For this review, take the finished solid that the model builds, in its own axes (mm). A direction names the side the tool comes from. Give positions to 0.01 mm unless a question says otherwise; leave off trailing zeros. Order: outer loops, then holes, each group sorted by start corner. A loop starts at its lowest first (then second) coordinate and runs counter-clockwise, first axis right, second up. Notation, with made-up numbers: (56, -2.5) - (66, -2.5) arc R12 ccw to (66, 8.5) - close; hole circle Ø3 at (36.5, 66.25). An arc over 180 degrees is marked (long way). One line per item, written item: value.
```python
from build123d import *

# Parameters (mm, degrees)
F0_W     = 76.2
F0_H     = 152.4
F1_DEPTH = 25.4
F2_W     = 33.02
F2_H     = 21.1666666667
F3_DEPTH = 22.86
F4_DEPTH = 22.86
F5_DEPTH = 22.86


# Not quite as in the source:
# - a feature names something its author has since deleted; it is built from what else it names


with BuildPart() as f1:
    # F0 (on Front) → F1 (new body)
    with BuildSketch(Plane.XZ):
        Rectangle(F0_W, F0_H)
    extrude(amount=F1_DEPTH)

    # F2 (on face) → F3 (cut)
    with BuildSketch(Plane.XZ.offset(25.4)):
        with Locations((-18.2778849706, 54.3725310351)):
            Rectangle(F2_W, F2_H)
    extrude(amount=-F3_DEPTH, mode=Mode.SUBTRACT)

    # F2 (on face) → F4 (cut)
    with BuildSketch(Plane.XZ.offset(25.4)):
        with Locations((19.8221150294, 54.3725310351)):
            Rectangle(F2_W, F2_H)
        with Locations((-19.05, 28.5166088839)):
            Rectangle(F2_W, F2_H)
        with Locations((-18.5682759488, -3.211494873)):
            Rectangle(F2_W, F2_H)
        with Locations((19.5317240512, -3.211494873)):
            Rectangle(F2_W, F2_H)
    extrude(amount=-F4_DEPTH, mode=Mode.SUBTRACT)

    # F2 (on face) → F5 (cut)
    with BuildSketch(Plane.XZ.offset(25.4)):
        with Locations((19.05, 28.5166088839)):
            Rectangle(F2_W, F2_H)
    extrude(amount=-F5_DEPTH, mode=Mode.SUBTRACT)


solid = f1.part
```
(1) Wall thickness on line 1 (Z direction, x = -34, y = -11); line 2 (X direction, y = -9.25, z = 23); line 3 (X direction, y = -16, z = 6.5): over which ranges is each line inside the solid? List them lowest first. Write a range as from..to.
Answers below:
line 1: z = -76.2..-13.79, 7.37..17.93, 39.1..43.79, 64.96..76.2
line 2: x = -38.1..-35.56, -2.54..2.54, 35.56..38.1
line 3: x = -38.1..-35.08, -2.06..3.02, 36.04..38.1
(2) Take a section at C-C (x = 17). Write out the cut boundary in (y, z).
Answers below:
outline: (-25.4, -76.2) - (0, -76.2) - (0, 76.2) - (-25.4, 76.2) - (-25.4, 64.96) - (-2.54, 64.96) - (-2.54, 43.79) - (-25.4, 43.79) - (-25.4, 39.1) - (-2.54, 39.1) - (-2.54, 17.93) - (-25.4, 17.93) - (-25.4, 7.37) - (-2.54, 7.37) - (-2.54, -13.79) - (-25.4, -13.79) - close
(3) Take a section at A-A (y = -8.5). Write out the cut boundary in (x, z).
Answers below:
outline: (-38.1, -76.2) - (38.1, -76.2) - (38.1, 76.2) - (-38.1, 76.2) - close; hole (-35.56, 17.93) - (-2.54, 17.93) - (-2.54, 39.1) - (-35.56, 39.1) - close; hole (-35.08, -13.79) - (-2.06, -13.79) - (-2.06, 7.37) - (-35.08, 7.37) - close; hole (-34.79, 43.79) - (-1.77, 43.79) - (-1.77, 64.96) - (-34.79, 64.96) - close; hole (2.54, 17.93) - (35.56, 17.93) - (35.56, 39.1) - (2.54, 39.1) - close; hole (3.02, -13.79) - (36.04, -13.79) - (36.04, 7.37) - (3.02, 7.37) - close; hole (3.31, 43.79) - (36.33, 43.79) - (36.33, 64.96) - (3.31, 64.96) - close
(4) Draft analysis for pull direction Z (two halves, no side actions). For faces 1 (the face through (-1, 0, 1)), 2 (the face through (35.56, -14, 28)), state which applies: pulls with the +Z half, pulls with the -Z half, needs draft (parallel to the pull), parting line crosses it, or undercut.
Answers below:
face 1: needs draft
face 2: undercut
(5) Take a section at B-B (z = 46). Write out the cut boundary in (x, y).
Answers below:
outline: (-38.1, -25.4) - (-34.79, -25.4) - (-34.79, -2.54) - (-1.77, -2.54) - (-1.77, -25.4) - (3.31, -25.4) - (3.31, -2.54) - (36.33, -2.54) - (36.33, -25.4) - (38.1, -25.4) - (38.1, 0) - (-38.1, 0) - close
(6) For P1, Ø6.5, axis at x = 19, z = 50.5, coming from the -Y side, flat-tipped, find the tip position at first contact; note if it passes through.
Answers below:
P1: stops at y = -2.54
(7) Machinability: for faces 3 (the face through (-19, -2.54, 29)), 4 (the face through (38.1, -13, -1)), which of the approach directions +Z, -Z, +X, -X, +Y, -Y give a long, thin tool a straight path to every point of the face, cutting with its end or side? Answer none if there is none.
Answers below:
face 3: -Y
face 4: +Z, -Z, +X, +Y, -Y
